```python
from build123d import *

# Parameters (mm, degrees)
PAD_DEPTH       = 8.85
SKETCH001_R     = 2.6
POCKET_DEPTH    = 78.001
SKETCH002_R     = 2.6
POCKET001_DEPTH = 78.001


with BuildPart() as part:
    # Sketch → Pad (new body, symmetric)
    with BuildSketch(Plane.XY):
        Polygon((0, 78), (0, 0), (78, 0), (78, 8), (30, 8), (8, 30), (8, 78), align=None)
    extrude(amount=PAD_DEPTH, both=True)

    # Sketch001 → Pocket (cut, through all)
    with BuildSketch(Plane.XZ):
        with Locations((39.65, 0)):
            Circle(SKETCH001_R)
        with Locations((68, 0)):
            Circle(SKETCH001_R)
    extrude(amount=-POCKET_DEPTH, mode=Mode.SUBTRACT)

    # Sketch002 → Pocket001 (cut, through all)
    with BuildSketch(Plane.YZ):
        with Locations((39.65, 0)):
            Circle(SKETCH002_R)
        with Locations((68, 0)):
            Circle(SKETCH002_R)
    extrude(amount=POCKET001_DEPTH, mode=Mode.SUBTRACT)


solid = part.part
```
Read the model definition and answer for the solid it produces. Units are mm, in the model's axes. A direction names the side the tool comes from. Round coordinates to 2 decimals unless told otherwise and drop trailing zeros. Write each loop counter-clockwise with the first axis right and the second up, starting at its lowest first coordinate (ties: lowest second). Pieces come first, ordered by that corner, then holes. Notation, with made-up numbers: M -40,6 L -9,6 A18 ccw -9,23 Z; hole C 62,27.25 d10. An arc over 180 degrees is marked long. One line per item, written item: value.
Q1. Find section D-D on z = -4.75. Write down the section's boundary in (x, y).
Data:
outline: M 0,0 L 78,0 L 78,8 L 30,8 L 8,30 L 8,78 L 0,78 Z
Q2. Find section A-A on x = 39.65. Write down the section's boundary in (y, z), plus the area to 3 significant figures.
Data:
outline: M 0,-8.85 L 8,-8.85 L 8,-2.6 L 0,-2.6 Z; M 0,2.6 L 8,2.6 L 8,8.85 L 0,8.85 Z
area: 100 mm2
Q3. Straight lines are drawn through the part: line 1 (Y direction, x = 5, z = 0); line 2 (Z direction, x = 3.5, y = 68); line 3 (X direction, y = 73, z = -7.5). For each, find the intervals that lie inside material, in ascending order. Write a range as [from, to].
Data:
line 1: [0, 37.05], [42.25, 65.4], [70.6, 78]
line 2: [-8.85, -2.6], [2.6, 8.85]
line 3: [0, 8]
Q4. Find section B-B on z = 0. Write down the section's boundary in (x, y).
Data:
outline: M 0,0 L 37.05,0 L 37.05,8 L 30,8 L 8,30 L 8,37.05 L 0,37.05 Z; M 0,42.25 L 8,42.25 L 8,65.4 L 0,65.4 Z; M 0,70.6 L 8,70.6 L 8,78 L 0,78 Z; M 42.25,0 L 65.4,0 L 65.4,8 L 42.25,8 Z; M 70.6,0 L 78,0 L 78,8 L 70.6,8 Z
Q5. Which of the six approach directions +Z, -Z, +X, -X, +Y, -Y give full straight-line access (tool end or side, diameter ignored) to faces 5 (the cylindrical face through (37.734, 3.944, 1.757)), 6 (the flat face through (54, 8, 0))?
Data:
face 5: +Y, -Y
face 6: +Z, -Z, +X, +Y
Q6. Flat-ended cylindrical pins translate along their axes: pin 1 Ø1.5 at (y, z) = (61.5, 0) entering from +X; pin 2 Ø4 at (x, z) = (43.5, 0.5) entering from +Y; pin 3 Ø1 at (y, z) = (20.5, -5) entering from +X. Find the tip coordinate at first contact, or state that the pin passes through.
Data:
pin 1: x = 8
pin 2: y = 8
pin 3: x = 18
Q7. For a pull along Z with two mould halves and no side action, classify faces 1 (the cylindrical face through (3.9, 65.4, 0.1)), 2 (the flat face through (4, 78, 0)), 3 (the flat face through (15.7, 21.8, -8.85)), 4 (the cylindrical face through (3.944, 37.734, 1.757)) as +Z half, -Z half, draft (parallel to the pull), parting line (faces both ways), or undercut.
Data:
face 1: undercut
face 2: draft
face 3: -Z half
face 4: undercut
